Geometry check sheet. Reference: the model listing, model coordinates, mm. A direction names the side the tool comes from. Round coordinates to 2 decimals unless told otherwise and drop trailing zeros. Write each loop counter-clockwise with the first axis right and the second up, starting at its lowest first coordinate (ties: lowest second). Pieces come first, ordered by that corner, then holes. Notation, with made-up numbers: (29.5, 8) - (56.5, 8) arc R30 cw to (56.5, 37) - close; hole circle Ø7 at (29, -17). An arc over 180 degrees is marked (long way). Return JSON: item names as keys, results as strings.
```python
from build123d import *

# Parameters (mm, degrees)
SKETCH_1_R          = 9.52
SKETCH_1_R_2        = 1.25
EXTRUDE_1_DEPTH     = 2
SKETCH_2_R          = 2.05
SKETCH_2_R_2        = 3.1
CUT_EXTRUDE_1_DEPTH = 4
FILLET_1_R          = 2
FILLET_3_R          = 30
FILLET_6_R          = 10


with BuildPart() as part:
    # 草图1 → 凸台-拉伸1 (new body)
    with BuildSketch(Plane.XY):
        with BuildLine():
            Line((328.542857143, -40.145714286), (-1.457142857, -40.145714286))
            Line((-1.457142857, -40.145714286), (-7.409980895, -22.36200829))
            ThreePointArc((-7.409980895, -22.36200829), (-24.457142857, -0.145714286), (-7.409980895, 22.070579719))
            Line((-7.409980895, 22.070579719), (-1.457142857, 39.854285714))
            Line((-1.457142857, 39.854285714), (75.684411109, 39.854285714))
            Line((75.684411109, 39.854285714), (85.544413109, 61.154285714))
            Line((85.544413109, 61.154285714), (96.174870529, 61.154285714))
            Line((96.174870529, 61.154285714), (106.145912956, 39.854285714))
            Line((106.145912956, 39.854285714), (321.071621128, 39.854285714))
            Line((321.071621128, 39.854285714), (328.542857143, 39.854285714))
            Line((328.542857143, 39.854285714), (334.49569518, 22.070579719))
            ThreePointArc((334.49569518, 22.070579719), (351.542857143, -0.145714286), (334.49569518, -22.36200829))
            Line((334.49569518, -22.36200829), (328.542857143, -40.145714286))
        make_face()
        with Locations((-1.457142857, -0.145714286)):
            Circle(SKETCH_1_R, mode=Mode.SUBTRACT)
        with Locations((328.542857143, -0.145714286)):
            Circle(SKETCH_1_R, mode=Mode.SUBTRACT)
        with Locations((318.542857143, 32.854285714)):
            Circle(SKETCH_1_R_2, mode=Mode.SUBTRACT)
        with BuildLine():
            ThreePointArc((318.542857143, 22.154285714), (326.108899702, 25.288243156), (329.242857143, 32.854285714))
            ThreePointArc((329.242857143, 32.854285714), (328.042857143, 34.054285714), (326.842857143, 32.854285714))
            ThreePointArc((326.842857143, 32.854285714), (324.411843427, 26.98529943), (318.542857143, 24.554285714))
            ThreePointArc((318.542857143, 24.554285714), (317.342857143, 23.354285714), (318.542857143, 22.154285714))
        make_face(mode=Mode.SUBTRACT)
    extrude(amount=EXTRUDE_1_DEPTH)

    # 草图2 → 切除-拉伸1 (cut)
    with BuildSketch(Plane.XY.offset(2)):
        with Locations((108.542857143, 33.854285714)):
            Circle(SKETCH_2_R)
        with Locations((198.542857143, 33.854285714)):
            Circle(SKETCH_2_R)
        with Locations((108.542857143, -34.145714286)):
            Circle(SKETCH_2_R)
        with Locations((198.542857143, -34.145714286)):
            Circle(SKETCH_2_R)
        with Locations((18.542857143, -34.145714286)):
            Circle(SKETCH_2_R)
        with Locations((18.542857143, 33.854285714)):
            Circle(SKETCH_2_R)
        with Locations((288.542857143, 33.854285714)):
            Circle(SKETCH_2_R_2)
        with Locations((288.542857143, -34.145714286)):
            Circle(SKETCH_2_R_2)
        Polygon((31.542857143, -21.145714286), (104.183898028, -21.145714286), (159.772133322, 20.854285714), (31.542857143, 20.854285714), align=None)
        Polygon((147.313580964, -21.145714286), (202.901816258, 20.854285714), (282.737923896, 20.854285714), (301.563806249, -0.145714286), (282.737923896, -21.145714286), align=None)
    extrude(amount=-CUT_EXTRUDE_1_DEPTH, mode=Mode.SUBTRACT)

    # 圆角1
    fillet_1_edges = [part.edges().sort_by_distance(p)[0] for p in [
        (282.737923896, -21.145714286, 1),
        (147.313580964, -21.145714286, 1),
        (202.901816258, 20.854285714, 1),
        (282.737923896, 20.854285714, 1),
        (301.563806249, -0.145714286, 1),
        (31.542857143, -21.145714286, 1),
        (31.542857143, 20.854285714, 1),
        (159.772133322, 20.854285714, 1),
        (104.183898028, -21.145714286, 1),
    ]]
    fillet(fillet_1_edges, radius=FILLET_1_R)

    # 圆角3
    # the kernel refuses this fillet: 30 mm, written as the material it takes off along each edge
    with BuildSketch(Plane(origin=(328.542857143, -40.145714286, -53.618003483), x_dir=(0.3174242162824087, 0.9482836426499714, 0), z_dir=(0, 0, 1))) as fillet_3_piece_1:
        with BuildLine():
            CenterArc((21.640648186, 29.86075675), FILLET_3_R, 198.507223716, 65.970321092)
            Line((-6.807861094, 20.338030262), (-7.376831279, 20.147575732))
            Line((-7.376831279, 20.147575732), (-0.568970186, -0.19045453))
            Line((-0.568970186, -0.19045453), (0, -0.6))
            ThreePointArc((0, -0.6), (9.376786225, -0.6), (18.695830935, -0.597215135))
            Line((18.695830935, -0.597215135), (18.75357245, 0))
        make_face()
    extrude(amount=109.236006966, mode=Mode.SUBTRACT)

    # 圆角6
    fillet_6_edges = [part.edges().sort_by_distance(p)[0] for p in [
        (328.542857143, 39.854285714, 1),
    ]]
    fillet(fillet_6_edges, radius=FILLET_6_R)


solid = part.part
```
(1) Release check for a two-part mould opening along X. For faces 1 (the face through (327.257, 37.919, 1.014)), 2 (the face through (80.545, 50.355, 0.986)), 3 (the face through (291.731, 10.822, 1.014)) record: pulls with the +X half, pulls with the -X half, needs draft (parallel to the pull), parting line crosses it, or undercut.
Response values:
{"face 1": "pulls with the +X half", "face 2": "pulls with the -X half", "face 3": "undercut"}
(2) Material ranges on line 1 along X through (y, z) = (14.5, 0.3); line 2 along X through (y, z) = (-3.5, 0.45); line 3 along X through (y, z) = (-8, 1.8), recorded low to high. Write a range as [from, to].
Response values:
{"line 1": "x = [-19.19, 31.54], [151.36, 194.49], [288.43, 346.28]", "line 2": "x = [-24.21, -10.37], [7.45, 31.54], [127.54, 170.67], [298.56, 319.63], [337.45, 351.3]", "line 3": "x = [-23.07, -6.84], [3.92, 31.54], [121.58, 164.71], [294.52, 323.16], [333.92, 350.16]"}
(3) Access from +Z, -Z, +X, -X, +Y, -Y to the whole of each face (thin tool, end or side, straight path). Record for faces 4 (the face through (326.03, 25.21, 0.99)), 5 (the face through (-24.453, -0.567, 0.986)).
Response values:
{"face 4": "+Z, -Z", "face 5": "+Z, -Z, -X"}
(4) Section check A-A, the plane x = 259. Enter the section's corners in (y, z).
Response values:
{"outline": "(-40.15, 0) - (-21.15, 0) - (-21.15, 2) - (-40.15, 2) - close; (20.85, 0) - (39.85, 0) - (39.85, 2) - (20.85, 2) - close"}
(5) Section check D-D, the plane z = 0.6. Give the number of separate pieces and of enclosed holes in the cut face, plus the area to 3 significant figures.
Response values:
{"separate pieces": "1", "enclosed holes": "14", "area": "18,700 mm^2"}
(6) Section check B-B, the plane x = 166. Enter the section's corners in (y, z), plus the area to 3 significant figures.
Response values:
{"outline": "(-40.15, 0) - (-21.15, 0) - (-21.15, 2) - (-40.15, 2) - close; (-7.03, 0) - (39.85, 0) - (39.85, 2) - (-7.03, 2) - close", "area": "132 mm^2"}
(7) Section check C-C, the plane y = 48. Enter the section's corners in (x, z), plus the area to 3 significant figures.
Response values:
{"outline": "(79.46, 0) - (102.33, 0) - (102.33, 2) - (79.46, 2) - close", "area": "45.8 mm^2"}
(8) Gauge pin test, flat end, axial feed: pin 1 (1 mm diameter, centred on x = 28, z = 1, fed in from +Y). Record the tip position at first contact, or that the pin passes through.
Response values:
{"pin 1": "stops at y = 39.85"}
